Geometry: final body of the model. Coordinates: model frame, mm. Give positions to 0.01 mm unless a question says otherwise; leave off trailing zeros. Order: outer loops, then holes, each group sorted by start corner. A loop starts at its lowest first (then second) coordinate and runs counter-clockwise, first axis right, second up. Notation, with made-up numbers: M -18.75,68.5 L -7.75,68.5 A19 cw -7.75,102.5 Z; hole C 49,-2.75 d5. An arc over 180 degrees is marked long. Use CSV: the item, a comma, the result in double quotes.
```python
from build123d import *

# Parameters (mm, degrees)
EXTRUDE_1_DEPTH     = 1
SKETCH_3_R          = 1.6
CUT_EXTRUDE_1_DEPTH = 10


with BuildPart() as part:
    # 草图2 → 凸台-拉伸1 (new body)
    with BuildSketch(Plane(origin=(0, 0, 0), x_dir=(1, 0, 0), z_dir=(0, 1, 0))):
        with BuildLine():
            Line((0, -47), (0, 47))
            Line((0, 47), (54, 47))
            Line((54, 47), (54, 42))
            ThreePointArc((54, 42), (23.114877049, 0), (54, -42))
            Line((54, -42), (54, -47))
            Line((54, -47), (0, -47))
        make_face()
    extrude(amount=EXTRUDE_1_DEPTH)

    # 草图3 → 切除-拉伸1 (cut)
    with BuildSketch(Plane(origin=(0, 1, 0), x_dir=(1, 0, 0), z_dir=(0, 1, 0))):
        with Locations(Location((15.5, 44, 0), (0, 0, 270))):
            Circle(SKETCH_3_R)
        with Locations(Location((35.5, 44, 0), (0, 0, 270))):
            Circle(SKETCH_3_R)
        with Locations(Location((15.5, -44, 0), (0, 0, 270))):
            Circle(SKETCH_3_R)
        with Locations(Location((35.5, -44, 0), (0, 0, 270))):
            Circle(SKETCH_3_R)
    extrude(amount=-CUT_EXTRUDE_1_DEPTH, mode=Mode.SUBTRACT)


solid = part.part
```
1. Line query: line 1 (X direction, y = 0.3, z = -44); line 2 (Z direction, x = 36.5, y = 0.7); line 3 (Z direction, x = 28, y = 0.7). Output: solid intervals per line, ascending.
Answer:
line 1,"0 to 13.9, 17.1 to 33.9, 37.1 to 54"
line 2,"-47 to -45.25, -42.75 to -31.6, 31.6 to 42.75, 45.25 to 47"
line 3,"-47 to -20.15, 20.15 to 47"
2. Pull-direction query (Z, two-part tool) for faces 1 (the face through (21, 1, -1)), 2 (the face through (34.08, 0.51, -43.26)); classes: +Z half, -Z half, draft (parallel to the pull), parting line (faces both ways), or undercut.
Answer:
face 1,"draft"
face 2,"undercut"
3. Pin query (flat end, axial travel): pin 1 Ø3 at (x, z) = (15.5, -44) entering from +Y. Return the tip coordinate at first contact, or that it passes through.
Answer:
pin 1,"through"
4. Section A-A, the plane z = 44. Return the cut outline in (x, y), plus the area to 3 significant figures.
Answer:
outline,"M 0,0 L 13.9,0 L 13.9,1 L 0,1 Z; M 17.1,0 L 33.9,0 L 33.9,1 L 17.1,1 Z; M 37.1,0 L 54,0 L 54,1 L 37.1,1 Z"
area,"47.6 mm2"
5. Section C-C, the plane y = 0.75. Return the cut outline in (x, z).
Answer:
outline,"M 0,-47 L 54,-47 L 54,-42 A44 cw 54,42 L 54,47 L 0,47 Z; hole C 15.5,-44 d3.2; hole C 15.5,44 d3.2; hole C 35.5,-44 d3.2; hole C 35.5,44 d3.2"
6. Section B-B, the plane x = 28.5. Return the cut outline in (y, z), plus the area to 3 significant figures.
Answer:
outline,"M 0,-47 L 1,-47 L 1,-21.09 L 0,-21.09 Z; M 0,21.09 L 1,21.09 L 1,47 L 0,47 Z"
area,"51.8 mm2"
7. Section D-D, the plane x = 35.5. Return the cut outline in (y, z), plus the area to 3 significant figures.
Answer:
outline,"M 0,-47 L 1,-47 L 1,-45.6 L 0,-45.6 Z; M 0,-42.4 L 1,-42.4 L 1,-30.6 L 0,-30.6 Z; M 0,30.6 L 1,30.6 L 1,42.4 L 0,42.4 Z; M 0,45.6 L 1,45.6 L 1,47 L 0,47 Z"
area,"26.4 mm2"
